from build123d import *

# Parameters (mm, degrees)
F0_R     = 30.15
F1_DEPTH = 18
F3_R     = 24.61
F4_DEPTH = 6
F5_R     = 5.99999
F6_R     = 10.65
F7_DEPTH = 25


# Not quite as in the source:
# - a fillet or chamfer is up to 0.001 mm smaller than in the source, because OpenCascade refuses the exact size


with BuildPart() as f1:
    # F0 (on Front) → F1 (new body)
    with BuildSketch(Plane.XZ):
        Circle(F0_R)
    extrude(amount=F1_DEPTH)

    # F3 (on face) → F4 (cut)
    with BuildSketch(Plane.XZ.offset(18)):
        Circle(F3_R)
    extrude(amount=-F4_DEPTH, mode=Mode.SUBTRACT)

    # F5 (radius 6 in the source; OpenCascade refuses exactly that, so slightly less here)
    f5_edges = [f1.edges().sort_by_distance(p)[0] for p in [
        (-24.61, -12, 0),
    ]]
    fillet(f5_edges, radius=F5_R)

    # F6 (on face) → F7 (cut)
    with BuildSketch(Plane.XZ.offset(18)):
        Circle(F6_R)
    extrude(amount=-F7_DEPTH, mode=Mode.SUBTRACT)

    # F8 (on Top) → F9 (revolve, cut)
    with BuildSketch(Plane.XY):
        Polygon((-30.15, -18.1521177292), (-25.61, -18), (-30.15, -14.5163354746), align=None)
    revolve(axis=Axis((0, -3.379675094, 0), (0, -1, 0)), mode=Mode.SUBTRACT)


solid = f1.part
Work out the finished part from the listing and answer in its coordinate system (mm). Give positions to 0.01 mm unless a question says otherwise; leave off trailing zeros. Write each loop counter-clockwise with the first axis right and the second up, starting at its lowest first coordinate (ties: lowest second). Pieces come first, ordered by that corner, then holes. Notation, with made-up numbers: (70, 29) - (77, 29) arc R30 cw to (77, 58) - close; hole circle Ø2 at (58, 29). An arc over 180 degrees is marked (long way). One line per item, written item: value. Start each with the question number.
1. Consider probe 1 along Z at (x, y) = (0, -7.5); probe 2 along Y at (x, z) = (12, -4); probe 3 along X at (y, z) = (-1, -6.5). Determine where each line is inside the solid, lowest interval first.
2. Find section C-C (y = -17). Write down the section's boundary in (x, z).
3. For a pull along X with two mould halves and no side action, classify faces 1 (the flat face through (-21, -18, 13.4)), 2 (the flat face through (8, -12, -8)), 3 (the conical face through (5.61, -17.78, 25.28)) as +X half, -X half, draft (parallel to the pull), parting line (faces both ways), or undercut.
4. Given pin 1 (24.5 mm diameter, centred on x = 0, z = 0, fed in from -Y); pin 2 (4 mm diameter, centred on x = -2, z = 21, fed in from +Y); pin 3 (3 mm diameter, centred on y = -9.5, z = -21, fed in from +X); pin 4 (3 mm diameter, centred on y = -10, z = -17, fed in from -X), each flat-ended and moving along its own axis, determine where each tip first touches the part or whether it passes through.
Geometry results:
1. probe 1: -30.15 to -10.65, 10.65 to 30.15
1. probe 2: -12 to 0
1. probe 3: -29.44 to -8.44, 8.44 to 29.44
2. outline: circle Ø53.83 at (0, 0); hole circle Ø49.05 at (0, 0)
3. face 1: draft
3. face 2: undercut
3. face 3: parting line
4. pin 1: y = -12
4. pin 2: y = 0
4. pin 3: x = 23
4. pin 4: x = -25.86
